Can you work these out from the drawing? Everything is in mm from the part's minimum corner. Round coordinates to 2 decimals unless told otherwise and drop trailing zeros. Write each loop counter-clockwise with the first axis right and the second up, starting at its lowest first coordinate (ties: lowest second). Pieces come first, ordered by that corner, then holes. Notation, with made-up numbers: (-12.5, 29) - (10.5, 29) arc R10 cw to (10.5, 34) - close; hole circle Ø6 at (6, 71). An arc over 180 degrees is marked (long way). One line per item, written item: value. Start each with the question number.
Item 1: If I drill on line 1 (X direction, y = 45, z = 3.05); line 2 (Y direction, x = 25, z = 0.85); line 3 (Z direction, x = 29.5, y = 25), over which ranges is the centre line in solid material (lowest first)?
Item 2: Thinking about a two-plate mould opening in Y: for the marked faces 1 and 2, which applies, released by +Y, released by -Y, zero draft, split by the parting line, or undercut?
Item 3: For P1, Ø1.5, axis at x = 26.5, y = 20.5, coming from the -Z side; P2, Ø3, axis at y = 5.5, z = 2.5, coming from the -X side; P3, Ø1.5, axis at x = 55.5, z = 2.5, coming from the -Y side, each with a flat end and sliding along its axis, tell me the tip position at first contact or that it passes through.
Item 4: Imagine slicing it at A-A, the plane x = 24. Please give me the cut outline in (y, z), then the cut area to 3 significant figures.
Item 5: Imagine slicing it at C-C, the plane y = 35. Please give me the cut outline in (x, z).
Item 6: Imagine slicing it at B-B, the plane z = 3.35. Please give me the cut outline in (x, y), then the cut area to 3 significant figures.
Item 7: Imagine slicing it at D-D, the plane x = 46. Please give me the cut outline in (y, z).
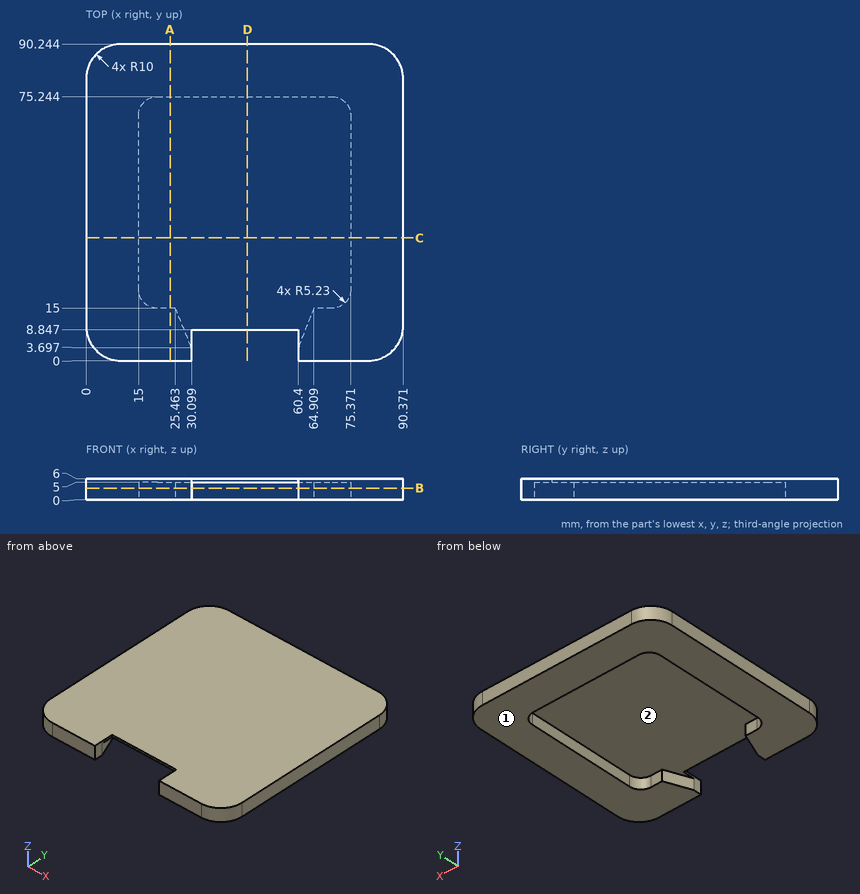
Values follow:
1. line 1: x = 0 to 15, 75.37 to 90.37
1. line 2: y = 0 to 15, 75.24 to 90.24
1. line 3: z = 5 to 6
2. face 1: zero draft
2. face 2: undercut
3. P1: stops at z = 5
3. P2: stops at x = 0.46
3. P3: stops at y = 75.24
4. outline: (0, 0) - (15, 0) - (15, 5) - (75.24, 5) - (75.24, 0) - (90.24, 0) - (90.24, 6) - (0, 6) - close
4. area: 240 mm^2
5. outline: (0, 0) - (15, 0) - (15, 5) - (75.37, 5) - (75.37, 0) - (90.37, 0) - (90.37, 6) - (0, 6) - close
6. outline: (0, 10) arc R10 ccw to (10, 0) - (30.1, 0) - (30.1, 3.7) - (25.46, 15) - (20.23, 15) arc R5.23 cw to (15, 20.23) - (15, 70.01) arc R5.23 cw to (20.23, 75.24) - (70.14, 75.24) arc R5.23 cw to (75.37, 70.01) - (75.37, 20.23) arc R5.23 cw to (70.14, 15) - (64.91, 15) - (60.4, 3.7) - (60.4, 0) - (80.37, 0) arc R10 ccw to (90.37, 10) - (90.37, 80.24) arc R10 ccw to (80.37, 90.24) - (10, 90.24) arc R10 ccw to (0, 80.24) - close
6. area: 3,950 mm^2
7. outline: (8.85, 5) - (75.24, 5) - (75.24, 0) - (90.24, 0) - (90.24, 6) - (8.85, 6) - close
